from build123d import *

# Parameters (mm, degrees)
BOSS_EXTRUDE1_DEPTH = 100
BOSS_EXTRUDE2_DEPTH = 2.5
SKETCH4_R           = 5
BOSS_EXTRUDE3_DEPTH = 7
SKETCH4_3_R         = 5.125
CUT_EXTRUDE1_DEPTH  = 7
SKETCH7_W           = 3.75
SKETCH7_H           = 8
CUT_EXTRUDE4_DEPTH  = 145


with BuildPart() as part:
    # Sketch2 → Boss-Extrude1 (new body)
    with BuildSketch(Plane.XY):
        Polygon((0, 0), (10, 0), (10, 20), (2.5, 20), (2.5, 10), (0, 10), align=None)
    boss_extrude1 = extrude(amount=BOSS_EXTRUDE1_DEPTH)

    # Sketch3 → Boss-Extrude2 (add)
    with BuildSketch(Plane.ZY.offset(-2.5)):
        with BuildLine():
            Line((1.919611614, 19.598058068), (0, 10))
            Line((0, 10), (5, 10))
            Line((5, 10), (3.080388386, 19.598058068))
            ThreePointArc((3.080388386, 19.598058068), (2.907092501, 19.886671071), (2.590098049, 20))
            Line((2.590098049, 20), (2.409901951, 20))
            ThreePointArc((2.409901951, 20), (2.092907499, 19.886671071), (1.919611614, 19.598058068))
        make_face()
        with BuildLine():
            Line((6.919611614, 19.598058068), (5, 10))
            Line((5, 10), (10, 10))
            Line((10, 10), (8.080388386, 19.598058068))
            ThreePointArc((8.080388386, 19.598058068), (7.907092501, 19.886671071), (7.590098049, 20))
            Line((7.590098049, 20), (7.409901951, 20))
            ThreePointArc((7.409901951, 20), (7.092907499, 19.886671071), (6.919611614, 19.598058068))
        make_face()
        with BuildLine():
            Line((11.919611614, 19.598058068), (10, 10))
            Line((10, 10), (15, 10))
            Line((15, 10), (13.080388386, 19.598058068))
            ThreePointArc((13.080388386, 19.598058068), (12.907092501, 19.886671071), (12.590098049, 20))
            Line((12.590098049, 20), (12.409901951, 20))
            ThreePointArc((12.409901951, 20), (12.092907499, 19.886671071), (11.919611614, 19.598058068))
        make_face()
        with BuildLine():
            Line((16.919611614, 19.598058068), (15, 10))
            Line((15, 10), (20, 10))
            Line((20, 10), (18.080388386, 19.598058068))
            ThreePointArc((18.080388386, 19.598058068), (17.907092501, 19.886671071), (17.590098049, 20))
            Line((17.590098049, 20), (17.409901951, 20))
            ThreePointArc((17.409901951, 20), (17.092907499, 19.886671071), (16.919611614, 19.598058068))
        make_face()
        with BuildLine():
            Line((21.919611614, 19.598058068), (20, 10))
            Line((20, 10), (25, 10))
            Line((25, 10), (23.080388386, 19.598058068))
            ThreePointArc((23.080388386, 19.598058068), (22.907092501, 19.886671071), (22.590098049, 20))
            Line((22.590098049, 20), (22.409901951, 20))
            ThreePointArc((22.409901951, 20), (22.092907499, 19.886671071), (21.919611614, 19.598058068))
        make_face()
        with BuildLine():
            Line((26.919611614, 19.598058068), (25, 10))
            Line((25, 10), (30, 10))
            Line((30, 10), (28.080388386, 19.598058068))
            ThreePointArc((28.080388386, 19.598058068), (27.907092501, 19.886671071), (27.590098049, 20))
            Line((27.590098049, 20), (27.409901951, 20))
            ThreePointArc((27.409901951, 20), (27.092907499, 19.886671071), (26.919611614, 19.598058068))
        make_face()
        with BuildLine():
            Line((31.919611614, 19.598058068), (30, 10))
            Line((30, 10), (35, 10))
            Line((35, 10), (33.080388386, 19.598058068))
            ThreePointArc((33.080388386, 19.598058068), (32.907092501, 19.886671071), (32.590098049, 20))
            Line((32.590098049, 20), (32.409901951, 20))
            ThreePointArc((32.409901951, 20), (32.092907499, 19.886671071), (31.919611614, 19.598058068))
        make_face()
        with BuildLine():
            Line((36.919611614, 19.598058068), (35, 10))
            Line((35, 10), (40, 10))
            Line((40, 10), (38.080388386, 19.598058068))
            ThreePointArc((38.080388386, 19.598058068), (37.907092501, 19.886671071), (37.590098049, 20))
            Line((37.590098049, 20), (37.409901951, 20))
            ThreePointArc((37.409901951, 20), (37.092907499, 19.886671071), (36.919611614, 19.598058068))
        make_face()
        with BuildLine():
            Line((41.919611614, 19.598058068), (40, 10))
            Line((40, 10), (45, 10))
            Line((45, 10), (43.080388386, 19.598058068))
            ThreePointArc((43.080388386, 19.598058068), (42.907092501, 19.886671071), (42.590098049, 20))
            Line((42.590098049, 20), (42.409901951, 20))
            ThreePointArc((42.409901951, 20), (42.092907499, 19.886671071), (41.919611614, 19.598058068))
        make_face()
        with BuildLine():
            Line((46.919611614, 19.598058068), (45, 10))
            Line((45, 10), (50, 10))
            Line((50, 10), (48.080388386, 19.598058068))
            ThreePointArc((48.080388386, 19.598058068), (47.907092501, 19.886671071), (47.590098049, 20))
            Line((47.590098049, 20), (47.409901951, 20))
            ThreePointArc((47.409901951, 20), (47.092907499, 19.886671071), (46.919611614, 19.598058068))
        make_face()
        with BuildLine():
            Line((51.919611614, 19.598058068), (50, 10))
            Line((50, 10), (55, 10))
            Line((55, 10), (53.080388386, 19.598058068))
            ThreePointArc((53.080388386, 19.598058068), (52.907092501, 19.886671071), (52.590098049, 20))
            Line((52.590098049, 20), (52.409901951, 20))
            ThreePointArc((52.409901951, 20), (52.092907499, 19.886671071), (51.919611614, 19.598058068))
        make_face()
        with BuildLine():
            Line((56.919611614, 19.598058068), (55, 10))
            Line((55, 10), (60, 10))
            Line((60, 10), (58.080388386, 19.598058068))
            ThreePointArc((58.080388386, 19.598058068), (57.907092501, 19.886671071), (57.590098049, 20))
            Line((57.590098049, 20), (57.409901951, 20))
            ThreePointArc((57.409901951, 20), (57.092907499, 19.886671071), (56.919611614, 19.598058068))
        make_face()
        with BuildLine():
            Line((61.919611614, 19.598058068), (60, 10))
            Line((60, 10), (65, 10))
            Line((65, 10), (63.080388386, 19.598058068))
            ThreePointArc((63.080388386, 19.598058068), (62.907092501, 19.886671071), (62.590098049, 20))
            Line((62.590098049, 20), (62.409901951, 20))
            ThreePointArc((62.409901951, 20), (62.092907499, 19.886671071), (61.919611614, 19.598058068))
        make_face()
        with BuildLine():
            Line((66.919611614, 19.598058068), (65, 10))
            Line((65, 10), (70, 10))
            Line((70, 10), (68.080388386, 19.598058068))
            ThreePointArc((68.080388386, 19.598058068), (67.907092501, 19.886671071), (67.590098049, 20))
            Line((67.590098049, 20), (67.409901951, 20))
            ThreePointArc((67.409901951, 20), (67.092907499, 19.886671071), (66.919611614, 19.598058068))
        make_face()
        with BuildLine():
            Line((71.919611614, 19.598058068), (70, 10))
            Line((70, 10), (75, 10))
            Line((75, 10), (73.080388386, 19.598058068))
            ThreePointArc((73.080388386, 19.598058068), (72.907092501, 19.886671071), (72.590098049, 20))
            Line((72.590098049, 20), (72.409901951, 20))
            ThreePointArc((72.409901951, 20), (72.092907499, 19.886671071), (71.919611614, 19.598058068))
        make_face()
        with BuildLine():
            Line((76.919611614, 19.598058068), (75, 10))
            Line((75, 10), (80, 10))
            Line((80, 10), (78.080388386, 19.598058068))
            ThreePointArc((78.080388386, 19.598058068), (77.907092501, 19.886671071), (77.590098049, 20))
            Line((77.590098049, 20), (77.409901951, 20))
            ThreePointArc((77.409901951, 20), (77.092907499, 19.886671071), (76.919611614, 19.598058068))
        make_face()
        with BuildLine():
            Line((81.919611614, 19.598058068), (80, 10))
            Line((80, 10), (85, 10))
            Line((85, 10), (83.080388386, 19.598058068))
            ThreePointArc((83.080388386, 19.598058068), (82.907092501, 19.886671071), (82.590098049, 20))
            Line((82.590098049, 20), (82.409901951, 20))
            ThreePointArc((82.409901951, 20), (82.092907499, 19.886671071), (81.919611614, 19.598058068))
        make_face()
        with BuildLine():
            Line((86.919611614, 19.598058068), (85, 10))
            Line((85, 10), (90, 10))
            Line((90, 10), (88.080388386, 19.598058068))
            ThreePointArc((88.080388386, 19.598058068), (87.907092501, 19.886671071), (87.590098049, 20))
            Line((87.590098049, 20), (87.409901951, 20))
            ThreePointArc((87.409901951, 20), (87.092907499, 19.886671071), (86.919611614, 19.598058068))
        make_face()
        with BuildLine():
            Line((96.919611614, 19.598058068), (95, 10))
            Line((95, 10), (100, 10))
            Line((100, 10), (98.080388386, 19.598058068))
            ThreePointArc((98.080388386, 19.598058068), (97.907092501, 19.886671071), (97.590098049, 20))
            Line((97.590098049, 20), (97.409901951, 20))
            ThreePointArc((97.409901951, 20), (97.092907499, 19.886671071), (96.919611614, 19.598058068))
        make_face()
        with BuildLine():
            Line((90, 10), (91.919611614, 19.598058068))
            ThreePointArc((91.919611614, 19.598058068), (92.092907499, 19.886671071), (92.409901951, 20))
            Line((92.409901951, 20), (92.590098049, 20))
            ThreePointArc((92.590098049, 20), (92.907092501, 19.886671071), (93.080388386, 19.598058068))
            Line((93.080388386, 19.598058068), (95, 10))
            Line((95, 10), (90, 10))
        make_face()
    boss_extrude2 = extrude(amount=BOSS_EXTRUDE2_DEPTH)

    # Mirror1: Boss-Extrude1, Boss-Extrude2 across plane
    add(boss_extrude1.mirror(Plane(origin=(0, 10, 100), x_dir=(0, 0, 1), z_dir=(1, 0, 0))))
    add(boss_extrude2.mirror(Plane(origin=(0, 10, 100), x_dir=(0, 0, 1), z_dir=(1, 0, 0))))

    # Sketch4 → Boss-Extrude3 (add)
    with BuildSketch(Plane.XZ):
        with Locations((0, 102.5)):
            Circle(SKETCH4_R)
    extrude(amount=-BOSS_EXTRUDE3_DEPTH)

    # Sketch4<3> → Cut-Extrude1 (cut)
    with BuildSketch(Plane.XZ):
        with Locations((0, 2.5)):
            Circle(SKETCH4_3_R)
    extrude(amount=-CUT_EXTRUDE1_DEPTH, mode=Mode.SUBTRACT)

    # Sketch7 → Cut-Extrude4 (cut)
    with BuildSketch(Plane(origin=(0, 0, 0), x_dir=(-1, 0, 0), z_dir=(0, 0, -1))):
        with Locations((-8.125, 9.5)):
            Rectangle(SKETCH7_W, SKETCH7_H)
        with Locations((8.125, 9.5)):
            Rectangle(SKETCH7_W, SKETCH7_H)
    extrude(amount=-CUT_EXTRUDE4_DEPTH, mode=Mode.SUBTRACT)


solid = part.part
Part model, mm, in its own coordinate system. Coordinates: 2 decimals unless noted, no trailing zeros. Write each loop counter-clockwise with the first axis right and the second up, starting at its lowest first coordinate (ties: lowest second). Pieces come first, ordered by that corner, then holes. Notation, with made-up numbers: (-5, -12) - (6, -12) arc R22 cw to (6, 19) - close; hole circle Ø6 at (63.5, 21). An arc over 180 degrees is marked (long way). Put each result on its own line as item: value.
1. Two-plate mould, pull along Z, no slides. Class faces 1 (the flat face through (-10, 3, 49)), 2 (the flat face through (0, 15, 99)), 3 (the flat face through (0, 15, 69)): +Z half, -Z half, draft (parallel to the pull), parting line (faces both ways), or undercut.
Final values:
face 1: draft
face 2: +Z half
face 3: undercut
2. Band-saw the part on D-D (z = 102.5). Write the cut outline in (x, y), then the cut area to 3 significant figures.
Final values:
outline: (-5, 0) - (5, 0) - (5, 7) - (-5, 7) - close
area: 70.0 mm²
3. Band-saw the part on B-B (y = 1.5). Write the cut outline in (x, z) (3 decimals), then the cut area to 3 significant figures.
Final values:
outline: (-10, 0) - (-4.474, 0) arc R5.125 cw (long way) to (4.474, 0) - (10, 0) - (10, 100) - (4.33, 100) arc R5 ccw (long way) to (-4.33, 100) - (-10, 100) - close
area: 2,000 mm²
4. Flat gauge pins, fed straight in: pin 1 Ø2 at (x, y) = (-1, 3.5) entering from -Z; pin 2 Ø6 at (x, y) = (0, 15.5) entering from +Z. Where does each tip first touch, or does it go through?
Final values:
pin 1: stops at z = 7.22
pin 2: stops at z = 100
5. Band-saw the part on A-A (z = 86). Write the cut outline in (x, y).
Final values:
outline: (-10, 0) - (10, 0) - (10, 5.5) - (6.25, 5.5) - (6.25, 13.5) - (10, 13.5) - (10, 20) - (2.5, 20) - (2.5, 15) - (-2.5, 15) - (-2.5, 20) - (-10, 20) - (-10, 13.5) - (-6.25, 13.5) - (-6.25, 5.5) - (-10, 5.5) - close
6. Probe line 1 along X through (y, z) = (3.5, 2.5) (3 decimals); line 2 along Y through (x, z) = (9.25, 80.5); line 3 along X through (y, z) = (17.5, 14). List the from-to ranges inside material, lowest first. Write a range as [from, to].
Final values:
line 1: x = [-10, -5.125], [5.125, 10]
line 2: y = [0, 5.5], [13.5, 20]
line 3: x = [-10, -2.5], [2.5, 10]
7. Band-saw the part on C-C (y = 12.5). Give the number of separate pieces and of enclosed holes in the cut face, then the cut area to 3 significant figures.
Final values:
separate pieces: 1
enclosed holes: 19
area: 1,150 mm²
